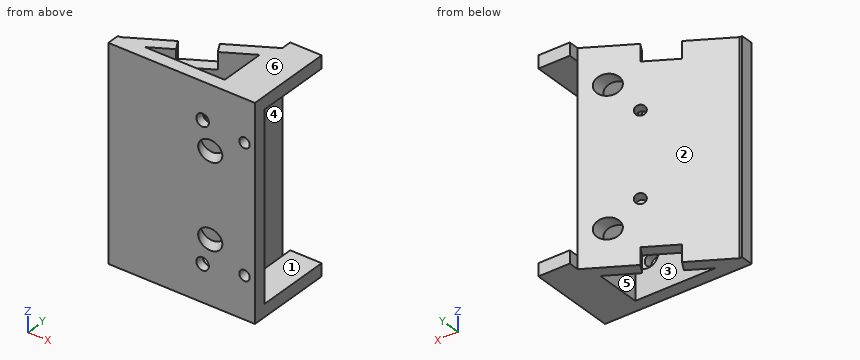
```python
from build123d import *

# Parameters (mm, degrees)
SKETCH1_W                      = 35
SKETCH1_H                      = 50
BOSS_EXTRUDE1_DEPTH            = 3
SKETCH2_R                      = 1.5
SKETCH2_R_2                    = 1.25
CUT_EXTRUDE1_DEPTH             = 4
BOSS_EXTRUDE2_DEPTH            = 50
CUT_EXTRUDE5_DEPTH             = 51
SKETCH8_R                      = 2.5
CUT_EXTRUDE6_DEPTH             = 16.5
CUT_EXTRUDE6_DEPTH_BACK        = 1
CUT_EXTRUDE7_REACH             = 21.771
SKETCH9_R                      = 1.25
SKETCH10_R                     = 2.5
CUT_EXTRUDE8_DEPTH             = 0.5
CUT_EXTRUDE8_DIRECTION_2_REACH = 18.874
SKETCH11_W                     = 7.5
SKETCH11_H                     = 3
BOSS_EXTRUDE3_DEPTH            = 18
CUT_EXTRUDE9_REACH             = 21.771
SKETCH14_W                     = 8
SKETCH14_H                     = 4


with BuildPart() as part:
    # Sketch1 → Boss-Extrude1 (new body)
    with BuildSketch(Plane(origin=(0, 0, 0), x_dir=(1, 0, 0), z_dir=(0, 1, 0))):
        with Locations((-87.623418825, 48.010907537)):
            Rectangle(SKETCH1_W, SKETCH1_H)
    extrude(amount=BOSS_EXTRUDE1_DEPTH)

    # Sketch2 → Cut-Extrude1 (cut, through all)
    with BuildSketch(Plane(origin=(0, 3, 0), x_dir=(1, 0, 0), z_dir=(0, 1, 0))):
        with Locations((-82.623418825, 64.263988227)):
            Circle(SKETCH2_R)
        with Locations((-82.623418825, 31.763988227)):
            Circle(SKETCH2_R)
        with Locations((-72.623418825, 33.010907537)):
            Circle(SKETCH2_R_2)
        with Locations((-72.623418825, 63.010907537)):
            Circle(SKETCH2_R_2)
    extrude(amount=-CUT_EXTRUDE1_DEPTH, mode=Mode.SUBTRACT)

    # Sketch4 → Boss-Extrude2 (add)
    with BuildSketch(Plane.XY.offset(-23.010907537)):
        Polygon((-77.623418825, 3), (-104.470206342, 3), (-77.623418825, 18.5), align=None)
    extrude(amount=-BOSS_EXTRUDE2_DEPTH)

    # Sketch6 → Cut-Extrude5 (cut, through all)
    with BuildSketch(Plane.XY.offset(-23.010907537)):
        Polygon((-98.675977708, 3), (-79.623418825, 3), (-79.623418825, 14), align=None)
    extrude(amount=-CUT_EXTRUDE5_DEPTH, mode=Mode.SUBTRACT)

    # Sketch8 → Cut-Extrude6 (cut, two sides)
    with BuildSketch(Plane(origin=(0, 3, 0), x_dir=(1, 0, 0), z_dir=(0, 1, 0))) as cut_extrude6_sk:
        with Locations((-82.623418825, 31.763988227)):
            Circle(SKETCH8_R)
        with Locations((-82.623418825, 64.263988227)):
            Circle(SKETCH8_R)
    extrude(amount=CUT_EXTRUDE6_DEPTH, mode=Mode.SUBTRACT)
    extrude(cut_extrude6_sk.sketch, amount=-CUT_EXTRUDE6_DEPTH_BACK, mode=Mode.SUBTRACT)

    # Sketch9 → Cut-Extrude7 (cut, up to next)
    with BuildSketch(Plane(origin=(-27.416589691, 47.486926315, 0), x_dir=(0.866025404, 0.5, 0), z_dir=(-0.5, 0.866025404, 0)), mode=Mode.PRIVATE) as cut_extrude7_sk1:
        with Locations((-69.973852631, 58.010907537)):
            Circle(SKETCH9_R)
    cut_extrude7_tool1 = extrude(cut_extrude7_sk1.sketch, amount=-CUT_EXTRUDE7_REACH, mode=Mode.PRIVATE) & part.part
    add(cut_extrude7_tool1.solids().sort_by_distance((-88.015724, 12.5, -58.010908))[0], mode=Mode.SUBTRACT)
    # Sketch9 → Cut-Extrude7 (cut, up to next)
    with BuildSketch(Plane(origin=(-27.416589691, 47.486926315, 0), x_dir=(0.866025404, 0.5, 0), z_dir=(-0.5, 0.866025404, 0)), mode=Mode.PRIVATE) as cut_extrude7_sk2:
        with Locations((-69.973852631, 38.010907537)):
            Circle(SKETCH9_R)
    cut_extrude7_tool2 = extrude(cut_extrude7_sk2.sketch, amount=-CUT_EXTRUDE7_REACH, mode=Mode.PRIVATE) & part.part
    add(cut_extrude7_tool2.solids().sort_by_distance((-88.015724, 12.5, -38.010908))[0], mode=Mode.SUBTRACT)

    # Sketch10 → Cut-Extrude8 (cut)
    with BuildSketch(Plane(origin=(-25.968032533, 44.977951719, 0), x_dir=(-0.866025404, -0.5, 0), z_dir=(0.5, -0.866025404, 0))):
        with Locations((69.973852631, 58.010907537)):
            Circle(SKETCH10_R)
        with Locations((69.973852631, 38.010907537)):
            Circle(SKETCH10_R)
    extrude(amount=-CUT_EXTRUDE8_DEPTH, mode=Mode.SUBTRACT)

    # Sketch10 → Cut-Extrude8 direction 2 (cut, up to next)
    with BuildSketch(Plane(origin=(-25.968032533, 44.977951719, 0), x_dir=(-0.866025404, -0.5, 0), z_dir=(0.5, -0.866025404, 0)), mode=Mode.PRIVATE) as cut_extrude8_direction_2_sk1:
        with Locations((69.973852631, 58.010907537)):
            Circle(SKETCH10_R)
    cut_extrude8_direction_2_tool1 = extrude(cut_extrude8_direction_2_sk1.sketch, amount=CUT_EXTRUDE8_DIRECTION_2_REACH, mode=Mode.PRIVATE) & part.part
    add(cut_extrude8_direction_2_tool1.solids().sort_by_distance((-86.567167, 9.991025, -58.010908))[0], mode=Mode.SUBTRACT)
    # Sketch10 → Cut-Extrude8 direction 2 (cut, up to next)
    with BuildSketch(Plane(origin=(-25.968032533, 44.977951719, 0), x_dir=(-0.866025404, -0.5, 0), z_dir=(0.5, -0.866025404, 0)), mode=Mode.PRIVATE) as cut_extrude8_direction_2_sk2:
        with Locations((69.973852631, 38.010907537)):
            Circle(SKETCH10_R)
    cut_extrude8_direction_2_tool2 = extrude(cut_extrude8_direction_2_sk2.sketch, amount=CUT_EXTRUDE8_DIRECTION_2_REACH, mode=Mode.PRIVATE) & part.part
    add(cut_extrude8_direction_2_tool2.solids().sort_by_distance((-86.567167, 9.991025, -38.010908))[0], mode=Mode.SUBTRACT)

    # Sketch11 → Boss-Extrude3 (add)
    with BuildSketch(Plane(origin=(0, 3, 0), x_dir=(1, 0, 0), z_dir=(0, 1, 0))):
        with Locations((-73.873418825, 24.510907537)):
            Rectangle(SKETCH11_W, SKETCH11_H)
        with Locations((-73.873418825, 71.510907537)):
            Rectangle(SKETCH11_W, SKETCH11_H)
    extrude(amount=BOSS_EXTRUDE3_DEPTH)

    # Sketch14 → Cut-Extrude9 (cut, up to next)
    with BuildSketch(Plane(origin=(-27.416589691, 47.486926315, 0), x_dir=(0.866025404, 0.5, 0), z_dir=(-0.5, 0.866025404, 0)), mode=Mode.PRIVATE) as cut_extrude9_sk1:
        with Locations((-73.973852631, 25.010907537)):
            Rectangle(SKETCH14_W, SKETCH14_H)
    cut_extrude9_tool1 = extrude(cut_extrude9_sk1.sketch, amount=-CUT_EXTRUDE9_REACH, mode=Mode.PRIVATE) & part.part
    add(cut_extrude9_tool1.solids().sort_by_distance((-91.479825, 10.5, -25.010908))[0], mode=Mode.SUBTRACT)
    # Sketch14 → Cut-Extrude9 (cut, up to next)
    with BuildSketch(Plane(origin=(-27.416589691, 47.486926315, 0), x_dir=(0.866025404, 0.5, 0), z_dir=(-0.5, 0.866025404, 0)), mode=Mode.PRIVATE) as cut_extrude9_sk2:
        with Locations((-73.973852631, 71.010907537)):
            Rectangle(SKETCH14_W, SKETCH14_H)
    cut_extrude9_tool2 = extrude(cut_extrude9_sk2.sketch, amount=-CUT_EXTRUDE9_REACH, mode=Mode.PRIVATE) & part.part
    add(cut_extrude9_tool2.solids().sort_by_distance((-91.479825, 10.5, -71.010908))[0], mode=Mode.SUBTRACT)


solid = part.part
```
Input: part model. Units: mm. Frame: model coordinates. Face numbers are marked on the shaded views. A direction names the side the tool comes from. Coordinates: 2 decimals unless noted, no trailing zeros. Write each loop counter-clockwise with the first axis right and the second up, starting at its lowest first coordinate (ties: lowest second). Pieces come first, ordered by that corner, then holes. Notation, with made-up numbers: (5, 2.5) -> (55, 2.5) arc R22 ccw to (55, 34.5) -> close; hole circle Ø5 at (0, -3). An arc over 180 degrees is marked (long way). Answer as a JSON object with one key per item and string values.
1. Section A-A on x = -91. Return the cut outline in (y, z).
Result set:
{"outline": "(0, -73.01) -> (3, -73.01) -> (3, -23.01) -> (0, -23.01) -> close; (7.43, -69.01) -> (10.78, -69.01) -> (10.78, -27.01) -> (7.43, -27.01) -> close"}
2. Access query for the marked faces 1, 2 and 3. Directions: +Z, -Z, +X, -X, +Y, -Y. A direction counts if a zero-diameter tool reaches every point of the face in a straight line with its end or side. Return the directions, or none.
Result set:
{"face 1": "+X, +Y", "face 2": "+Z, -Z, -X, +Y", "face 3": "+Z, -Z"}
3. Mould query, pull axis Z, two halves, no side actions, for the marked faces 4, 5 and 6. Classes: released by +Z, released by -Z, zero draft, split by the parting line, or undercut.
Result set:
{"face 4": "undercut", "face 5": "zero draft", "face 6": "released by +Z"}
4. Section D-D on x = -83. Count the separate pieces of the cut face and the enclosed holes in it, then the cut area to 3 significant figures.
Result set:
{"separate pieces": "8", "enclosed holes": "0", "area": "237 mm2"}
5. Section C-C on y = 16.25. Return the cut outline in (x, z), then the cut area to 3 significant figures.
Result set:
{"outline": "(-81.52, -73.01) -> (-70.12, -73.01) -> (-70.12, -70.01) -> (-77.62, -70.01) -> (-77.62, -26.01) -> (-70.12, -26.01) -> (-70.12, -23.01) -> (-81.52, -23.01) -> (-81.52, -29.52) arc R2.5 cw to (-81.52, -34.01) -> (-81.52, -62.02) arc R2.5 cw to (-81.52, -66.51) -> close", "area": "231 mm2"}
6. Section B-B on y = 7.5. Return the cut outline in (x, z).
Result set:
{"outline": "(-96.68, -73.01) -> (-94.37, -73.01) -> (-94.37, -69.01) -> (-90.88, -69.01) -> (-90.88, -27.01) -> (-94.37, -27.01) -> (-94.37, -23.01) -> (-96.68, -23.01) -> close; (-79.62, -73.01) -> (-70.12, -73.01) -> (-70.12, -70.01) -> (-77.62, -70.01) -> (-77.62, -26.01) -> (-70.12, -26.01) -> (-70.12, -23.01) -> (-79.62, -23.01) -> close"}
7. Material intervals for line 1 (Z direction, x = -77, y = 6.75); line 2 (X direction, y = 2.5, z = -32); line 3 (Y direction, x = -73, z = -68), sorted ascending. Write a range as from..to.
Result set:
{"line 1": "z = -73.01..-70.01, -26.01..-23.01", "line 2": "x = -105.12..-85.11, -80.13..-73.36, -71.89..-70.12", "line 3": "y = 0..3"}
8. First-contact query: P1, Ø3, axis at y = 17.5, z = -55, coming from the -X side; P2, Ø2, axis at x = -84, y = 5, coming from the +Z side; P3, Ø3.5, axis at x = -90.5, y = 11, coming from the +Z side; P4, Ø10, axis at x = -92, z = -38.5, coming from the +Y side. Flat tips, straight axial feed; report the tip coordinate or a pass-through.
Result set:
{"P1": "stops at x = -81.95", "P2": "passes through", "P3": "stops at z = -27.01", "P4": "stops at y = 13.09"}
